Can you work these out from the model? Positions are in its coordinate system, mm. Round coordinates to 2 decimals unless told otherwise and drop trailing zeros. Order: outer loops, then holes, each group sorted by start corner. A loop starts at its lowest first (then second) coordinate and runs counter-clockwise, first axis right, second up. Notation, with made-up numbers: (75, -29.5) -> (114, -29.5) arc R7 cw to (114, -16.5) -> close; hole circle Ø7 at (9.5, -27.5). An arc over 180 degrees is marked (long way). One line per item, written item: value.
```python
from build123d import *

# Parameters (mm, degrees)
SKETCH2_R           = 52.18
SKETCH2_R_2         = 4.075
BOSS_EXTRUDE2_DEPTH = 3.5
CUT_EXTRUDE1_DEPTH  = 2.5
SKETCH4_R           = 1.75
CUT_EXTRUDE2_DEPTH  = 146.860967066


with BuildPart() as part:
    # Sketch2 → Boss-Extrude2 (new body)
    with BuildSketch(Plane.XY):
        with Locations((-50.929581789, 50.929581789)):
            Circle(SKETCH2_R)
        with Locations((-50.929581789, 50.929581789)):
            Circle(SKETCH2_R_2, mode=Mode.SUBTRACT)
    extrude(amount=BOSS_EXTRUDE2_DEPTH)

    # Sketch3 → Cut-Extrude1 (cut)
    with BuildSketch(Plane.XY.offset(3.5)):
        Polygon((-53.729581789, 32.546162543), (-53.729581789, 29.313001036), (-50.929581789, 27.696420282), (-48.129581789, 29.313001036), (-48.129581789, 32.546162543), (-50.929581789, 34.162743297), align=None)
        Polygon((-32.546162543, 48.129581789), (-29.313001036, 48.129581789), (-27.696420282, 50.929581789), (-29.313001036, 53.729581789), (-32.546162543, 53.729581789), (-34.162743297, 50.929581789), align=None)
        Polygon((-7.546162543, 48.129581789), (-4.313001036, 48.129581789), (-2.696420282, 50.929581789), (-4.313001036, 53.729581789), (-7.546162543, 53.729581789), (-9.162743297, 50.929581789), align=None)
        Polygon((-69.313001036, 53.729581789), (-72.546162543, 53.729581789), (-74.162743297, 50.929581789), (-72.546162543, 48.129581789), (-69.313001036, 48.129581789), (-67.696420282, 50.929581789), align=None)
        Polygon((-48.129581789, 69.313001036), (-48.129581789, 72.546162543), (-50.929581789, 74.162743297), (-53.729581789, 72.546162543), (-53.729581789, 69.313001036), (-50.929581789, 67.696420282), align=None)
        Polygon((-17.477457052, 23.164200178), (-14.861774446, 21.263795526), (-11.908134437, 22.578840784), (-11.570177034, 25.794290694), (-14.185859639, 27.694695347), (-17.139499648, 26.379650089), align=None)
        Polygon((-40.186326214, 8.804250632), (-39.187224362, 5.729331312), (-36.024715191, 5.057119236), (-33.861307871, 7.45982648), (-34.860409723, 10.5347458), (-38.022918894, 11.206957876), align=None)
        Polygon((-66.998753856, 10.5347458), (-67.997855708, 7.45982648), (-65.834448388, 5.057119236), (-62.671939216, 5.729331312), (-61.672837365, 8.804250632), (-63.836244685, 11.206957876), align=None)
        Polygon((-87.67330394, 27.694695347), (-90.288986545, 25.794290694), (-89.951029141, 22.578840784), (-86.997389132, 21.263795526), (-84.381706527, 23.164200178), (-84.719663931, 26.379650089), align=None)
        Polygon((-94.313001036, 53.729581789), (-97.546162543, 53.729581789), (-99.162743297, 50.929581789), (-97.546162543, 48.129581789), (-94.313001036, 48.129581789), (-92.696420282, 50.929581789), align=None)
        Polygon((-84.381706527, 78.694963401), (-86.997389132, 80.595368053), (-89.951029141, 79.280322795), (-90.288986545, 76.064872885), (-87.67330394, 74.164468232), (-84.719663931, 75.47951349), align=None)
        Polygon((-61.672837365, 93.054912947), (-62.671939216, 96.129832267), (-65.834448388, 96.802044343), (-67.997855708, 94.399337098), (-66.998753856, 91.324417778), (-63.836244685, 90.652205703), align=None)
        Polygon((-34.860409723, 91.324417778), (-33.861307871, 94.399337098), (-36.024715191, 96.802044343), (-39.187224362, 96.129832267), (-40.186326214, 93.054912947), (-38.022918894, 90.652205703), align=None)
        Polygon((-14.185859639, 74.164468232), (-11.570177034, 76.064872885), (-11.908134437, 79.280322795), (-14.861774446, 80.595368053), (-17.477457052, 78.694963401), (-17.139499648, 75.47951349), align=None)
    extrude(amount=-CUT_EXTRUDE1_DEPTH, mode=Mode.SUBTRACT)

    # Sketch4 → Cut-Extrude2 (cut, through all)
    with BuildSketch(Plane.XY.offset(3.5)):
        with Locations((-30.929581789, 50.929581789)):
            Circle(SKETCH4_R)
        with Locations((-5.929581789, 50.929581789)):
            Circle(SKETCH4_R)
        with Locations((-50.929581789, 30.929581789)):
            Circle(SKETCH4_R)
        with Locations((-70.929581789, 50.929581789)):
            Circle(SKETCH4_R)
        with Locations((-50.929581789, 70.929581789)):
            Circle(SKETCH4_R)
        with Locations((-14.523817043, 24.479245436)):
            Circle(SKETCH4_R)
        with Locations((-37.023817043, 8.132038556)):
            Circle(SKETCH4_R)
        with Locations((-64.835346536, 8.132038556)):
            Circle(SKETCH4_R)
        with Locations((-87.335346536, 24.479245436)):
            Circle(SKETCH4_R)
        with Locations((-95.929581789, 50.929581789)):
            Circle(SKETCH4_R)
        with Locations((-87.335346536, 77.379918143)):
            Circle(SKETCH4_R)
        with Locations((-64.835346536, 93.727125023)):
            Circle(SKETCH4_R)
        with Locations((-37.023817043, 93.727125023)):
            Circle(SKETCH4_R)
        with Locations((-14.523817043, 77.379918143)):
            Circle(SKETCH4_R)
    extrude(amount=-CUT_EXTRUDE2_DEPTH, mode=Mode.SUBTRACT)


solid = part.part
```
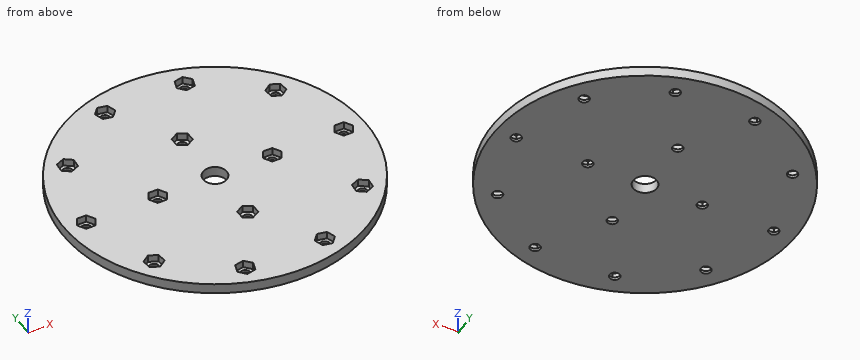
Q1. Please list where these lines run through material, in increasing order: line 1 along Y through (x, z) = (-50, 2.1); line 2 along X through (y, z) = (50, 2.05); line 3 along X through (y, z) = (9, 2).
Answers below:
line 1: -1.24 to 28.23, 33.63 to 46.96, 54.9 to 68.23, 73.63 to 103.1
line 2: -103.1 to -98.63, -93.23 to -73.63, -68.23 to -54.9, -46.96 to -33.63, -28.23 to -8.63, -3.23 to 1.24
line 3: -81.99 to -67.5, -61.85 to -40.01, -34.36 to -19.87
Q2. Will these pins go through, and if not, where does the flat tip stop? pin 1 Ø1 at (x, z) = (-75, 3) entering from +Y; pin 2 Ø4.5 at (x, y) = (-50, 30) entering from +Z; pin 3 Ø2 at (y, z) = (92, 2) entering from +X; pin 4 Ø0.8 at (x, z) = (-30.5, 2.5) entering from -Y.
Answers below:
pin 1: y = 97.48
pin 2: z = 3.5
pin 3: x = -17.51
pin 4: y = 2.75
Q3. I want a section at B-B on y = 15.5. List the corners of the cut face in (x, z) for me.
Answers below:
outline: (-89.24, 0) -> (-12.62, 0) -> (-12.62, 3.5) -> (-89.24, 3.5) -> close
Q4. I want a section at C-C on x = -19. List the corners of the cut face in (y, z) for me.
Answers below:
outline: (9.66, 0) -> (92.2, 0) -> (92.2, 3.5) -> (9.66, 3.5) -> close
Q5. I want a section at A-A on z = 1.55. Give the number of separate pieces and of enclosed holes in the cut face, plus the area to 3 significant figures.
Answers below:
separate pieces: 1
enclosed holes: 15
area: 8,120 mm^2
